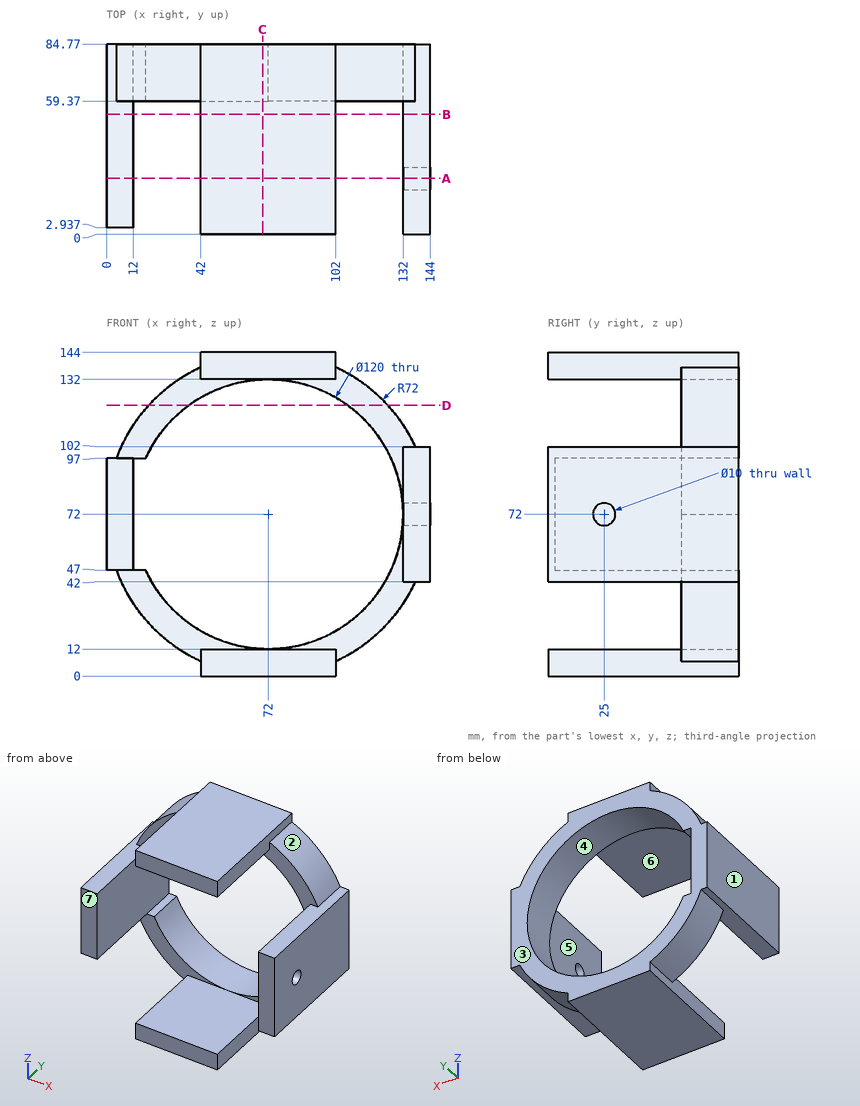
Input: dimensioned drawing with shaded views. Units: mm. Origin: part minimum x, y, z. A direction names the side the tool comes from. Round coordinates to 2 decimals unless told otherwise and drop trailing zeros. Loops run counter-clockwise (first coordinate to the right, second up) from the corner with the lowest first, then second, coordinate; pieces in that order, holes last. Notation, with made-up numbers: (68, 27.25) -> (80, 27.25) arc R17 cw to (80, 32.25) -> close; hole circle Ø8 at (12, -29). An arc over 180 degrees is marked (long way). Answer as a JSON object with one key per item and string values. Group by question number.
1) Section query D-D on z = 120.5. Output: boundary loops of the cut face in (x, y) (1 decimal).
2) Section query B-B on y = 53.5. Output: boundary loops of the cut face in (x, z).
3) Reachability of the marked faces 5, 6 and 7 from +Z, -Z, +X, -X, +Y, -Y: full face, straight path, thin tool, end or side. Return the list, or none.
4) Draft query along X for the marked faces 1, 2, 3 and 4. Return one class per face: +X half, -X half, draft (parallel to the pull), parting line (faces both ways), or undercut.
5) Pin query (flat end, axial travel): pin 1 (1 mm diameter, centred on y = 63.5, z = 24, fed in from +X); pin 2 (6 mm diameter, centred on x = 136.5, y = 45, fed in from -Z); pin 3 (4 mm diameter, centred on y = 73, z = 102, fed in from -X). Return the tip coordinate at first contact, or that it passes through.
6) Section query C-C on x = 69.5. Output: boundary loops of the cut face in (y, z), plus the area to 3 significant figures.
7) Ray query, L1, parallel to Y at x = 139.25, z = 72; L2, parallel to X at y = 12, z = 80. Return the intervals inside material, ascending.
8) Section query A-A on y = 25. Output: boundary loops of the cut face in (x, z), plus the area to 3 significant figures.
Reply:
{
 "1": {"outline": "(18.8, 59.4) -> (36.7, 59.4) -> (36.7, 84.8) -> (18.8, 84.8) -> close; (107.3, 59.4) -> (125.2, 59.4) -> (125.2, 84.8) -> (107.3, 84.8) -> close"},
 "2": {"outline": "(0, 47) -> (12, 47) -> (12, 97) -> (0, 97) -> close; (42, 0) -> (102, 0) -> (102, 12) -> (42, 12) -> close; (42, 132) -> (102, 132) -> (102, 144) -> (42, 144) -> close; (132, 42) -> (144, 42) -> (144, 102) -> (132, 102) -> close"},
 "3": {"face 5": "+Z, -Z, -Y", "face 6": "+X, -X, -Y", "face 7": "+Z, -Z, -X, -Y"},
 "4": {"face 1": "-X half", "face 2": "+X half", "face 3": "draft", "face 4": "undercut"},
 "5": {"pin 1": "stops at x = 126.11", "pin 2": "stops at z = 42", "pin 3": "stops at x = 5.67"},
 "6": {"outline": "(0, 0) -> (84.77, 0) -> (84.77, 12.05) -> (59.37, 12.05) -> (59.37, 12) -> (0, 12) -> close; (0, 132) -> (59.37, 132) -> (59.37, 131.95) -> (84.77, 131.95) -> (84.77, 144) -> (0, 144) -> close", "area": "2,040 mm2"},
 "7": {"L1": "y = 0 to 20, 30 to 84.77", "L2": "x = 0 to 12, 132 to 144"},
 "8": {"outline": "(0, 47) -> (12, 47) -> (12, 97) -> (0, 97) -> close; (42, 0) -> (102, 0) -> (102, 12) -> (42, 12) -> close; (42, 132) -> (102, 132) -> (102, 144) -> (42, 144) -> close; (132, 42) -> (144, 42) -> (144, 67) -> (132, 67) -> close; (132, 77) -> (144, 77) -> (144, 102) -> (132, 102) -> close", "area": "2,640 mm2"}
}
